Could you check a few things on this drawing? It's one solid part, dimensions in mm from its lowest x, y, z. Coordinates: 2 decimals unless noted, no trailing zeros. Order: outer loops, then holes, each group sorted by start corner. A loop starts at its lowest first (then second) coordinate and runs counter-clockwise, first axis right, second up. Notation, with made-up numbers: (65, -36.75) -> (78, -36.75) arc R25 ccw to (78, -20.75) -> close; hole circle Ø10 at (57.5, 64). An arc over 180 degrees is marked (long way). Use a Markdown table: item, result. Add a question column.
1. For pin 1 Ø4 at (y, z) = (4.5, 5) entering from -X; pin 2 Ø6 at (y, z) = (7, 13.5) entering from +X; pin 3 Ø3 at (y, z) = (16.5, 6) entering from +X, each with a flat end and sliding along its axis, tell me the tip position at first contact or that it passes through.
2. Suppose I cut it at C-C, the plane x = 93.5. List the corners of the cut face in (y, z) for me, then the cut area to 3 significant figures.
3. If I drill on line 1 along X through (y, z) = (10.5, 12.75); line 2 along Z through (x, y) = (90.5, 4); line 3 along X through (y, z) = (17.75, 8.5), over which ranges is the centre line in solid material (lowest first)? Write a range as from..to.
4. Suppose I cut it at A-A, the plane y = 8.25. List the corners of the cut face in (x, z) for me, then the cut area to 3 significant figures.
5. Suppose I cut it at B-B, the plane z = 7.5. List the corners of the cut face in (x, y) for me, then the cut area to 3 significant figures.
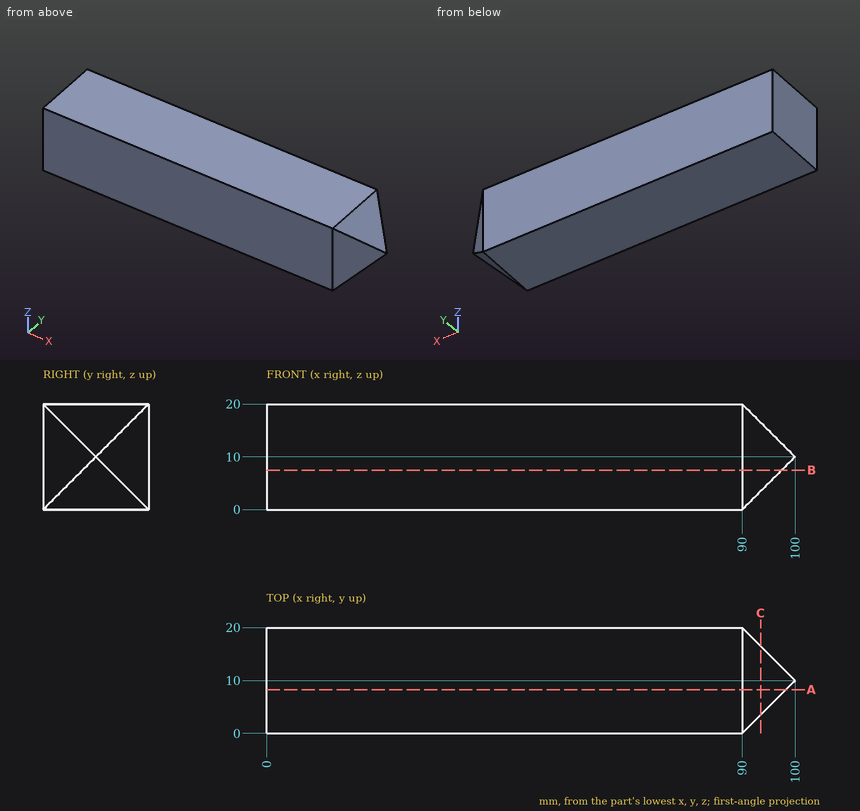
Worked out:
| question | item | result |
|---|---|---|
| 1 | pin 1 | stops at x = 0 |
| 1 | pin 2 | stops at x = 98.86 |
| 1 | pin 3 | stops at x = 95 |
| 2 | outline | (3.5, 3.5) -> (16.5, 3.5) -> (16.5, 16.5) -> (3.5, 16.5) -> close |
| 2 | area | 169 mm² |
| 3 | line 1 | x = 0..97.25 |
| 3 | line 2 | z = 0.5..19.5 |
| 3 | line 3 | x = 0..92.25 |
| 4 | outline | (0, 0) -> (90, 0) -> (98.25, 8.25) -> (98.25, 11.75) -> (90, 20) -> (0, 20) -> close |
| 4 | area | 1,900 mm² |
| 5 | outline | (0, 0) -> (90, 0) -> (97.5, 7.5) -> (97.5, 12.5) -> (90, 20) -> (0, 20) -> close |
| 5 | area | 1,890 mm² |
